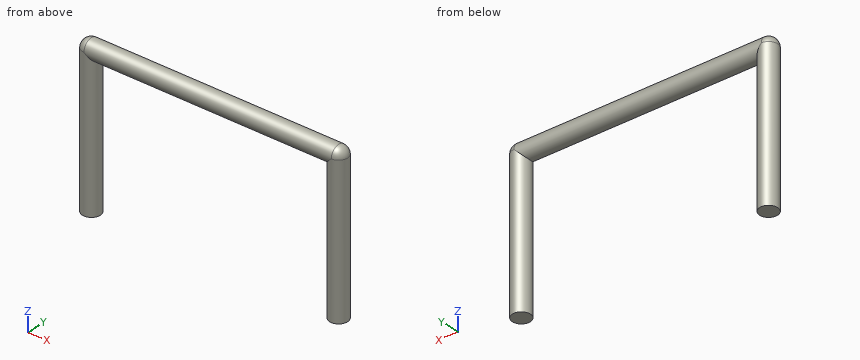
Autodesk Inventor part; units mm, degrees
sketch "Sketch1" plane through (0, 0, 0) normal (0, 0, 1) x (1, 0, 0)
  circle A0 centre (-5, 0) radius 0.3635
  circle A1 centre (5, 0) radius 0.3635
  line L0 (-7.5089, 0) -> (7.5089, 0)
  point P0 (0, 0)
  point P1 (-5.3635, 0)
  point P2 (-4.6365, 0)
  dimension "d2" = 0.727
  dimension "d3" = 0.727
  dimension "d4" = 10
  dimension "d5" = 5
extrude "Extrusion1" add sketch "Sketch1" along normal blind 6
sketch "Sketch2" plane through (0, 0, 0) normal (0, 1, 0) x (-1, 0, 0)
  line L0 (-4.6365, 6) -> (-5.3635, 6)
  circle A0 centre (-5, 6) radius 0.3635
  line L1 (5.3635, 6) -> (4.6365, 6)
  circle A1 centre (5, 6) radius 0.3635
  line L2 (5, 6.3635) -> (-5, 6.3635)
  line L3 (-5, 6) -> (5, 6)
  point P0 (0, 0)
revolve "Revolution1" add sketch "Sketch2" angle 360 about axis through (5, 0, 6) along (-1, 0, 0) picked at (-5.1703, 6.1703) picked at (4.8297, 6.1703) contours L0 A0 | A0 L2 A1 L3 | A1 L1
properties part number "Wire" material "S235"
Work out the finished part from the listing and answer in its coordinate system (mm). Coordinates: 2 decimals unless noted, no trailing zeros. Write each loop counter-clockwise with the first axis right and the second up, starting at its lowest first coordinate (ties: lowest second). Pieces come first, ordered by that corner, then holes. Notation, with made-up numbers: (-36.5, 30) - (-23.5, 30) arc R18 cw to (-23.5, 62) - close; hole circle Ø4 at (63, 64). An arc over 180 degrees is marked (long way). Answer as a JSON object with one key per item and string values.
Q1. Find section C-C (x = -1.75). Write down the section's boundary in (y, z).
Results list:
{"outline": "circle Ø0.73 at (0, 6)"}
Q2. Consider L1, parallel to X at y = -0.05, z = 3.5; L2, parallel to Z at x = -0.5, y = -0.05; L3, parallel to X at y = 0.2, z = 4.75. Determine where each line is inside the solid, lowest interval first. Write a range as from..to.
Results list:
{"L1": "x = -5.36..-4.64, 4.64..5.36", "L2": "z = 5.64..6.36", "L3": "x = -5.3..-4.7, 4.7..5.3"}
Q3. Find section A-A (z = 5.5). Write down the section's boundary in (x, y), plus the area to 3 significant figures.
Results list:
{"outline": "circle Ø0.73 at (-5, 0); circle Ø0.73 at (5, 0)", "area": "0.830 mm^2"}
Q4. Find section B-B (y = 0). Write down the section's boundary in (x, z), plus the area to 3 significant figures.
Results list:
{"outline": "(-5.36, 0) - (-4.64, 0) - (-4.64, 5.64) - (4.64, 5.64) - (4.64, 0) - (5.36, 0) - (5.36, 6) arc R0.36 ccw to (5, 6.36) - (-5, 6.36) arc R0.36 ccw to (-5.36, 6) - close", "area": "15.9 mm^2"}
